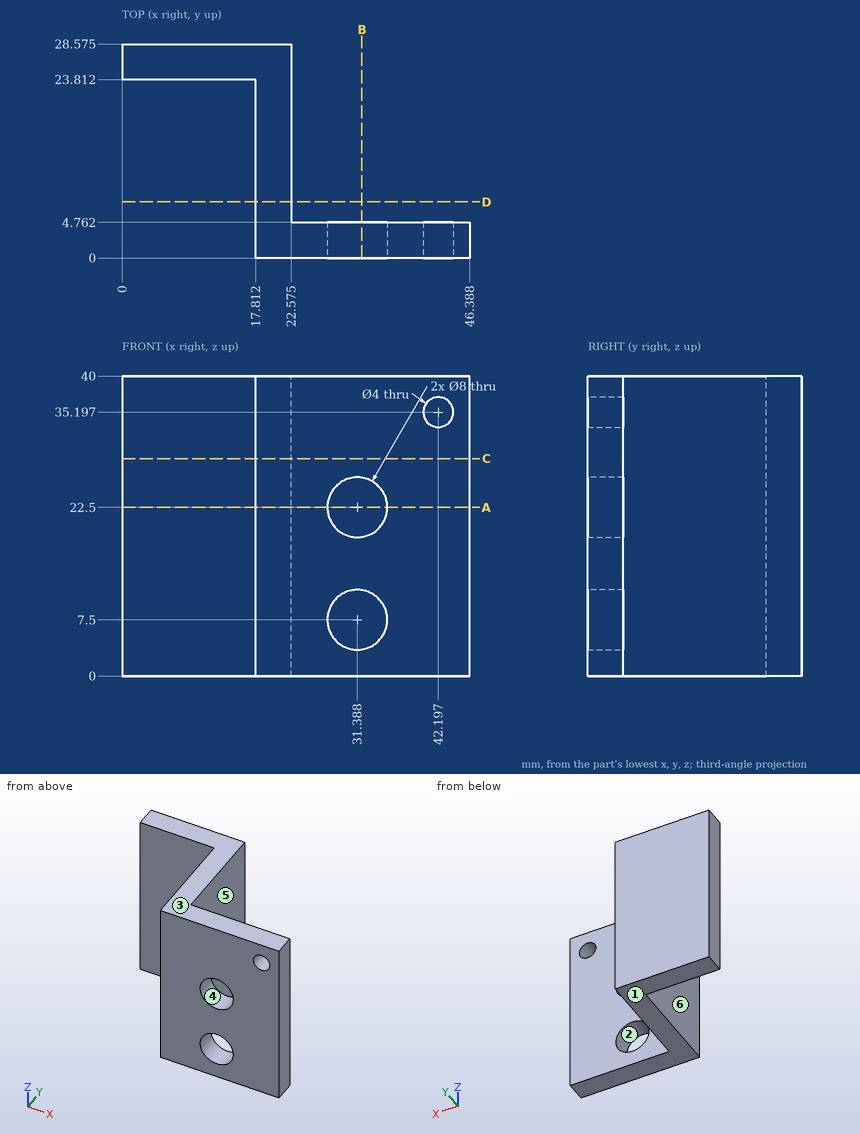
Geometry check sheet. Reference: drawing and pictorial views, mm from the part's lowest x, y, z. A direction names the side the tool comes from. Coordinates: 2 decimals unless noted, no trailing zeros. Order: outer loops, then holes, each group sorted by start corner. A loop starts at its lowest first (then second) coordinate and runs counter-clockwise, first axis right, second up.
Item 1: Tool access check on the marked faces 4, 5 and 6. Record the directions out of +Z, -Z, +X, -X, +Y, -Y that give a thin tool (end or side, any length) a straight path to the whole face; none if there is none.
Item 2: Section check D-D (y = 7.5). Enter the section's corners in (x, z) (1 decimal).
Item 3: Scan lines: line 1 along X through (y, z) = (3.2, 7.5); line 2 along Y through (x, z) = (16, 9.5) (1 decimal); line 3 along Y through (x, z) = (29, 38.5). Record each from-to range of solid material in increasing order.
Item 4: Section check C-C (z = 29). Enter the section's corners in (x, y) (1 decimal).
Item 5: Section check A-A (z = 22.5). Enter the section's corners in (x, y) (1 decimal), plus the area to 3 significant figures.
Item 6: Section check B-B (x = 32). Enter the section's corners in (y, z), plus the area to 3 significant figures.
Item 7: Mould release check, pull along Z, two halves, no side actions. Record for the marked faces 1, 2 and 3: released by +Z, released by -Z, zero draft, split by the parting line, or undercut.
Item 8: Depth check by flat-ended pin: pin 1 (5 mm diameter, centred on y = 16, z = 20, fed in from -X); pin 2 (2 mm diameter, centred on x = 33.5, z = 11.5, fed in from +Y); pin 3 (7 mm diameter, centred on x = 31.39, z = 7.5, fed in from +Y); pin 4 (10 mm diameter, centred on x = 15.5, y = 14, fed in from -Z). Enter the tip coordinate at first touch or a pass-through.
Check sheet entries:
1. face 4: +Y, -Y
1. face 5: +Z, -Z, +X, +Y
1. face 6: +Z, -Z, -X, -Y
2. outline: (17.8, 0) - (22.6, 0) - (22.6, 40) - (17.8, 40) - close
3. line 1: x = 17.81 to 27.39, 35.39 to 46.39
3. line 2: y = 23.8 to 28.6
3. line 3: y = 0 to 4.76
4. outline: (0, 23.8) - (17.8, 23.8) - (17.8, 0) - (46.4, 0) - (46.4, 4.8) - (22.6, 4.8) - (22.6, 28.6) - (0, 28.6) - close
5. outline: (0, 23.8) - (17.8, 23.8) - (17.8, 0) - (27.4, 0) - (27.4, 4.8) - (22.6, 4.8) - (22.6, 28.6) - (0, 28.6) - close; (35.4, 0) - (46.4, 0) - (46.4, 4.8) - (35.4, 4.8) - close
5. area: 296 mm2
6. outline: (0, 0) - (4.76, 0) - (4.76, 3.55) - (0, 3.55) - close; (0, 11.45) - (4.76, 11.45) - (4.76, 18.55) - (0, 18.55) - close; (0, 26.45) - (4.76, 26.45) - (4.76, 40) - (0, 40) - close
6. area: 115 mm2
7. face 1: released by -Z
7. face 2: undercut
7. face 3: released by +Z
8. pin 1: stops at x = 17.81
8. pin 2: stops at y = 4.76
8. pin 3: passes through
8. pin 4: stops at z = 0
